Source: CAD feature listing. Evaluate the final solid. Frame: model axes, mm. A direction names the side the tool comes from. Give positions to 0.01 mm unless a question says otherwise; leave off trailing zeros. Loops run counter-clockwise (first coordinate to the right, second up) from the corner with the lowest first, then second, coordinate; pieces in that order, holes last.
```python
from build123d import *

# Parameters (mm, degrees)
F2_W          = 37.102
F2_H          = 46.096
F2_W_2        = 30
F2_H_2        = 16
F3_DEPTH      = 27.4
F4_W          = 5.5
F4_H          = 8
F4_W_2        = 5
F5_DEPTH      = 5
F5_DEPTH_BACK = 13
F6_R          = 5.9111779492
F7_DEPTH      = 25
F8_W          = 25
F8_H          = 24.945173396
F9_DEPTH      = 10


with BuildPart() as f1:
    # F0 (on Front) → F1 (revolve)
    with BuildSketch(Plane.XZ):
        Polygon((-1.5167587905, -24.0440348498), (-0.4654595977, -24.895950213), (0, -24.895950213), (0, -5.4683293174), (0, 38.0978930385), (-8, 38.0978930385), (-8, 33.2978930385), (-6, 33.2978930385), (-6, 28.6978930385), (-8, 28.6978930385), (-8, 25.1978930385), (-6, 25.1978930385), (-6, 20.5978930385), (-15, 20.5978930385), (-15, -5.4021069615), (-2.5, -5.4021069615), (-2.5, -14.9021069615), (-4, -14.9021069615), (-4, -22.9021069615), (-1.9699050371, -22.9202326714), (-1.5167587905, -23.1921206525), align=None)
    revolve(axis=Axis((0, 0, 26.8247116869), (0, 0, 1)))

    # F2 (on face) → F3 (cut)
    with BuildSketch(Plane.XY.offset(20.5978930385)):
        Rectangle(F2_W, F2_H)
        Rectangle(F2_W_2, F2_H_2, mode=Mode.SUBTRACT)
    extrude(amount=-F3_DEPTH, mode=Mode.SUBTRACT)

    # F4 (on Front) → F5 (join, two sides)
    with BuildSketch(Plane.XZ) as f5_sk:
        Polygon((8, -6.812995024), (2.5, -6.812995024), (2.5, -14.812995024), (4, -14.812995024), (8, -14.812995024), align=None)
        with Locations((-5.25, -10.812995024)):
            Rectangle(F4_W, F4_H)
        with Locations((0, -10.812995024)):
            Rectangle(F4_W_2, F4_H)
    extrude(amount=F5_DEPTH)
    extrude(f5_sk.sketch, amount=-F5_DEPTH_BACK)

    # F6 (on face) → F7 (cut)
    with BuildSketch(Plane(origin=(0, 0, -14.812995024), x_dir=(1, 0, 0), z_dir=(0, 0, -1))):
        Circle(F6_R)
        Polygon((3.6810046325, -1.6683939069), (0.3956308093, -4.0220404767), (-3.2853738232, -2.3536465697), (-3.6810046325, 1.6683939069), (-0.3956308093, 4.0220404767), (3.2853738232, 2.3536465697), align=None, mode=Mode.SUBTRACT)
    extrude(amount=F7_DEPTH, mode=Mode.SUBTRACT)

    # F8 (on face) → F9 (join)
    with BuildSketch(Plane(origin=(0, 8, 0), x_dir=(-1, 0, 0), z_dir=(0, 1, 0))):
        with Locations((0, 7.0704797366)):
            Rectangle(F8_W, F8_H)
    extrude(amount=F9_DEPTH)


solid = f1.part
```
(1) Section D-D, the plane x = 5. Return the cut outline in (y, z) (3 decimals).
A:
outline: (-8, -5.402) - (18, -5.402) - (18, 19.543) - (8, 19.543) - (8, 20.598) - (3.317, 20.598) - (3.317, 25.198) - (6.245, 25.198) - (6.245, 28.698) - (3.317, 28.698) - (3.317, 33.298) - (6.245, 33.298) - (6.245, 38.098) - (-6.245, 38.098) - (-6.245, 33.298) - (-3.317, 33.298) - (-3.317, 28.698) - (-6.245, 28.698) - (-6.245, 25.198) - (-3.317, 25.198) - (-3.317, 20.598) - (-8, 20.598) - close; (-5, -14.813) - (13, -14.813) - (13, -6.813) - (-5, -6.813) - close
(2) Section C-C, the plane y = 4.75. Return the cut outline in (x, z), then the cut area to 3 significant figures.
A:
outline: (-14.23, -5.4) - (14.23, -5.4) - (14.23, 20.6) - (3.67, 20.6) - (3.67, 25.2) - (6.44, 25.2) - (6.44, 28.7) - (3.67, 28.7) - (3.67, 33.3) - (6.44, 33.3) - (6.44, 38.1) - (-6.44, 38.1) - (-6.44, 33.3) - (-3.67, 33.3) - (-3.67, 28.7) - (-6.44, 28.7) - (-6.44, 25.2) - (-3.67, 25.2) - (-3.67, 20.6) - (-14.23, 20.6) - close; (-8, -14.81) - (8, -14.81) - (8, -6.81) - (-8, -6.81) - close
area: 1,040 mm2
(3) Section B-B, the plane x = -9.75. Return the cut outline in (y, z).
A:
outline: (-8, -5.4) - (18, -5.4) - (18, 19.54) - (8, 19.54) - (8, 20.6) - (-8, 20.6) - close
(4) Section A-A, the plane z = 10.5. Return the cut outline in (x, y).
A:
outline: (-12.69, -8) - (12.69, -8) arc R15 ccw to (12.69, 8) - (12.5, 8) - (12.5, 18) - (-12.5, 18) - (-12.5, 8) - (-12.69, 8) arc R15 ccw to start
(5) Ray query, line 1 along Z through (x, y) = (-2.25, -6.5); line 2 along Z through (x, y) = (3, 9.75); line 3 along Z through (x, y) = (-4.5, 2). Return the intervals inside material, ascending.
A:
line 1: z = -5.4 to 20.6, 25.2 to 28.7, 33.3 to 38.1
line 2: z = -14.81 to -6.81, -5.4 to 19.54
line 3: z = -14.81 to -6.81, -5.4 to 38.1
(6) Mould query, pull axis Z, two halves, no side actions, for faces 6 (the cylindrical face through (15, 0, 7)), 7 (the cylindrical face through (6, 0, 23)), 8 (the flat face through (0, 0, 38.098)). Classes: pulls with the +Z half, pulls with the -Z half, needs draft (parallel to the pull), parting line crosses it, or undercut.
A:
face 6: needs draft
face 7: undercut
face 8: pulls with the +Z half
(7) First-contact query: pin 1 (3 mm diameter, centred on y = 11, z = 4.5, fed in from +X); pin 2 (2.5 mm diameter, centred on x = -4, z = -9.5, fed in from -Y); pin 3 (6.5 mm diameter, centred on y = 5, z = -11, fed in from -X); pin 4 (12 mm diameter, centred on x = 2.5, z = 28.5, fed in from -Y). Flat tips, straight axial feed; report the tip coordinate or a pass-through.
A:
pin 1: stops at x = 12.5
pin 2: stops at y = -5
pin 3: stops at x = -8
pin 4: stops at y = -8
(8) Reachability of faces 1 (the flat face through (2.1, 2.8, -18.8)), 2 (the cylindrical face through (1.73, 7.81, 26.92)), 3 (the flat face through (1.42, -3.2, -18.85)), 4 (the flat face through (-2.1, -2.8, -18.8)), 5 (the flat face through (12.5, 13, 7)) from +Z, -Z, +X, -X, +Y, -Y: full face, straight path, thin tool, end or side. Return the list, or none.
A:
face 1: -Z, +X, +Y
face 2: +Z
face 3: -Z, +X, -Y
face 4: -Z, -X, -Y
face 5: +Z, -Z, +X, +Y
